For this review, take the finished solid that the model builds, in its own axes (mm). Round coordinates to 2 decimals unless told otherwise and drop trailing zeros. Order: outer loops, then holes, each group sorted by start corner. A loop starts at its lowest first (then second) coordinate and runs counter-clockwise, first axis right, second up. Notation, with made-up numbers: (-4, 69) -> (30, 69) arc R15 cw to (30, 85) -> close; hole circle Ø11 at (47.25, -6). An arc over 180 degrees is marked (long way). Answer in a Markdown table with one row per item.
Autodesk Inventor part; units mm, degrees
ref_plane "YZ Plane" through (0, 0, 0) normal (1, 0, 0) x (0, 1, 0)
ref_plane "XZ Plane" through (0, 0, 0) normal (0, 1, 0) x (-1, 0, 0)
ref_plane "XY Plane" through (0, 0, 0) normal (0, 0, 1) x (1, 0, 0)
sketch "Sketch_5" plane through (0, 0, 0) normal (0, 0, 1) x (1, 0, 0)
  line L0 (-10, 9) -> (-10, 3.3)
  arc A0 (-10, 3.3) -> (-9.7, 3) centre (-9.7, 3.3) ccw
  line L1 (-9.7, 3) -> (-8, 3)
  line L2 (-8, 3) -> (-8, 6)
  line L3 (-8, 6) -> (-7.0607, 6)
  line L4 (-7.0607, 6) -> (-4, 2.9393)
  line L5 (-4, 2.9393) -> (-4, 0.3)
  line L6 (-4, 0.3) -> (-3.7, 0)
  line L7 (-3.7, 0) -> (-4, -0.3)
  line L8 (-4, -0.3) -> (-4, -2.9393)
  line L9 (-4, -2.9393) -> (-7.0607, -6)
  line L10 (-7.0607, -6) -> (-8, -6)
  line L11 (-8, -6) -> (-8, -3)
  line L12 (-8, -3) -> (-9.7, -3)
  arc A1 (-9.7, -3) -> (-10, -3.3) centre (-9.7, -3.3) ccw
  line L13 (-10, -3.3) -> (-10, -9)
  arc A2 (-10, -9) -> (-9, -10) centre (-9, -9) ccw
  line L14 (-9, -10) -> (-3.3, -10)
  arc A3 (-3.3, -10) -> (-3, -9.7) centre (-3.3, -9.7) ccw
  line L15 (-3, -9.7) -> (-3, -8)
  line L16 (-3, -8) -> (-6, -8)
  line L17 (-6, -8) -> (-6, -7.0607)
  line L18 (-6, -7.0607) -> (-2.9393, -4)
  line L19 (-2.9393, -4) -> (-0.3, -4)
  line L20 (-0.3, -4) -> (0, -3.7)
  line L21 (0, -3.7) -> (0.3, -4)
  line L22 (0.3, -4) -> (2.9393, -4)
  line L23 (2.9393, -4) -> (6, -7.0607)
  line L24 (6, -7.0607) -> (6, -8)
  line L25 (6, -8) -> (3, -8)
  line L26 (3, -8) -> (3, -9.7)
  arc A4 (3, -9.7) -> (3.3, -10) centre (3.3, -9.7) ccw
  line L27 (3.3, -10) -> (9, -10)
  arc A5 (9, -10) -> (10, -9) centre (9, -9) ccw
  line L28 (10, -9) -> (10, -3.3)
  arc A6 (10, -3.3) -> (9.7, -3) centre (9.7, -3.3) ccw
  line L29 (9.7, -3) -> (8, -3)
  line L30 (8, -3) -> (8, -6)
  line L31 (8, -6) -> (7.0607, -6)
  line L32 (7.0607, -6) -> (4, -2.9393)
  line L33 (4, -2.9393) -> (4, -0.3)
  line L34 (4, -0.3) -> (3.7, 0)
  line L35 (3.7, 0) -> (4, 0.3)
  line L36 (4, 0.3) -> (4, 2.9393)
  line L37 (4, 2.9393) -> (7.0607, 6)
  line L38 (7.0607, 6) -> (8, 6)
  line L39 (8, 6) -> (8, 3)
  line L40 (8, 3) -> (9.7, 3)
  arc A7 (9.7, 3) -> (10, 3.3) centre (9.7, 3.3) ccw
  line L41 (10, 3.3) -> (10, 9)
  arc A8 (10, 9) -> (9, 10) centre (9, 9) ccw
  line L42 (9, 10) -> (3.3, 10)
  arc A9 (3.3, 10) -> (3, 9.7) centre (3.3, 9.7) ccw
  line L43 (3, 9.7) -> (3, 8)
  line L44 (3, 8) -> (6, 8)
  line L45 (6, 8) -> (6, 7.0607)
  line L46 (6, 7.0607) -> (2.9393, 4)
  line L47 (2.9393, 4) -> (0.3, 4)
  line L48 (0.3, 4) -> (0, 3.7)
  line L49 (0, 3.7) -> (-0.3, 4)
  line L50 (-0.3, 4) -> (-2.9393, 4)
  line L51 (-2.9393, 4) -> (-6, 7.0607)
  line L52 (-6, 7.0607) -> (-6, 8)
  line L53 (-6, 8) -> (-3, 8)
  line L54 (-3, 8) -> (-3, 9.7)
  arc A10 (-3, 9.7) -> (-3.3, 10) centre (-3.3, 9.7) ccw
  line L55 (-3.3, 10) -> (-9, 10)
  arc A11 (-9, 10) -> (-10, 9) centre (-9, 9) ccw
  circle A12 centre (0, 0) radius 2.1
extrude "Extrusion1" add sketch "Sketch_5" against normal blind 51.5
properties part number "KHFS5-2020-4000"
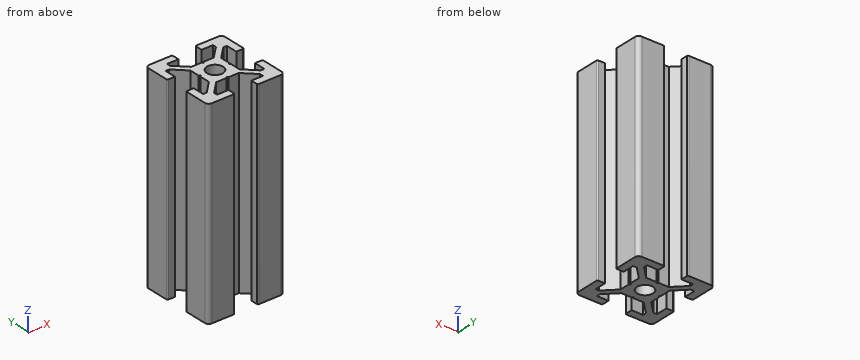
Q1. To check wall thickness, follow probe 1 along Y at (x, z) = (4.25, -12); probe 2 along Y at (x, z) = (4.5, -34); probe 3 along X at (y, z) = (5.75, -15). State the ranges of each line that lie inside material, in increasing order.
Answer key:
| item | result |
|---|---|
| probe 1 | y = -10 to -8, -5.31 to -3.19, 3.19 to 5.31, 8 to 10 |
| probe 2 | y = -10 to -8, -5.56 to -3.44, 3.44 to 5.56, 8 to 10 |
| probe 3 | x = -10 to -8, -6.81 to -4.69, 4.69 to 6.81, 8 to 10 |
Q2. Take a section at A-A, the plane y = 5.5. Write out the cut boundary in (x, z), then the cut area to 3 significant figures.
Answer key:
| item | result |
|---|---|
| outline | (-10, -51.5) -> (-8, -51.5) -> (-8, 0) -> (-10, 0) -> close; (-6.56, -51.5) -> (-4.44, -51.5) -> (-4.44, 0) -> (-6.56, 0) -> close; (4.44, -51.5) -> (6.56, -51.5) -> (6.56, 0) -> (4.44, 0) -> close; (8, -51.5) -> (10, -51.5) -> (10, 0) -> (8, 0) -> close |
| area | 425 mm^2 |
Q3. Take a section at B-B, the plane y = -1.25. Write out the cut boundary in (x, z).
Answer key:
| item | result |
|---|---|
| outline | (-4, -51.5) -> (-1.69, -51.5) -> (-1.69, 0) -> (-4, 0) -> close; (1.69, -51.5) -> (4, -51.5) -> (4, 0) -> (1.69, 0) -> close |
Q4. Clearance check with flat-ended pins moving along their axes: pin 1 Ø2 at (y, z) = (-1, -19) entering from -X; pin 2 Ø3 at (x, z) = (-0.5, -33) entering from +Y; pin 3 Ø0.8 at (x, z) = (2, -31.5) entering from -Y. State where each tip first meets the part, or that it passes through.
Answer key:
| item | result |
|---|---|
| pin 1 | stops at x = -4 |
| pin 2 | stops at y = 4 |
| pin 3 | stops at y = -4 |
